```python
from build123d import *

# Parameters (mm, degrees)
SZKIC1_W                    = 12.5
SZKIC1_H                    = 37
DODANIE_WYCI_GNI_CIE1_DEPTH = 9.9
SZKIC2_W                    = 6.3
SZKIC2_H                    = 23.2
WYTNIJ_WYCI_GNI_CIE1_DEPTH  = 9.9
SZKIC3_R                    = 2
SZKIC3_R_2                  = 3.65
DODANIE_WYCI_GNI_CIE2_DEPTH = 7.5
WYTNIJ_WYCI_GNI_CIE2_DEPTH  = 78.151879433
WYTNIJ_WYCI_GNI_CIE3_DEPTH  = 72.402310887
ESQUISSE2_W                 = 2.9
ESQUISSE2_H                 = 5.1
ENL_V_MAT_EXTRU_1_DEPTH     = 6.3
BOSS_EXTRU_2_START          = -2.5
ESQUISSE5_R                 = 3.65
BOSS_EXTRU_2_DEPTH          = 2.5
BOSS_EXTRU_3_DEPTH          = 37
ESQUISSE7_R                 = 1.1
BOSS_EXTRU_4_DEPTH          = 4.5
ESQUISSE8_R                 = 1.65
ESQUISSE8_R_2               = 1.1
ENL_V_MAT_EXTRU_2_DEPTH     = 2.3
BOSS_EXTRU_7_START          = 1.2
BOSS_EXTRU_7_DEPTH          = 1.2
ENL_V_MAT_EXTRU_3_DEPTH     = 75.421317511
ENL_V_MAT_EXTRU_4_DEPTH     = 75.088410025


with BuildPart() as part:
    # Szkic1 → Dodanie-wyciągnięcie1 (new body)
    with BuildSketch(Plane.XY):
        with Locations((-6.25, 18.5)):
            Rectangle(SZKIC1_W, SZKIC1_H)
    extrude(amount=DODANIE_WYCI_GNI_CIE1_DEPTH)

    # Szkic2 → Wytnij-wyciągnięcie1 (cut)
    with BuildSketch(Plane.XY.offset(9.9)):
        with Locations((-3.15, 18.5)):
            Rectangle(SZKIC2_W, SZKIC2_H)
    extrude(amount=-WYTNIJ_WYCI_GNI_CIE1_DEPTH, mode=Mode.SUBTRACT)

    # Szkic3 → Dodanie-wyciągnięcie2 (add)
    with BuildSketch(Plane.ZY.offset(12.5)):
        with BuildLine():
            Line((55.440769231, 18.25), (57.7, -4))
            ThreePointArc((57.7, -4), (51.55, -10.15), (45.4, -4))
            Line((45.4, -4), (45.4, 0))
            Line((45.4, 0), (7.4, 0))
            Line((7.4, 0), (7.4, 37))
            Line((7.4, 37), (9.9, 37))
            Line((9.9, 37), (55.440769231, 18.25))
        make_face()
        with Locations((51.55, 12.25)):
            Circle(SZKIC3_R, mode=Mode.SUBTRACT)
        with Locations((51.55, -4)):
            Circle(SZKIC3_R_2, mode=Mode.SUBTRACT)
    extrude(amount=DODANIE_WYCI_GNI_CIE2_DEPTH)

    # Szkic4 → Wytnij-wyciągnięcie2 (cut, through all)
    with BuildSketch(Plane(origin=(0, 37, 0), x_dir=(1, 0, 0), z_dir=(0, 1, 0))):
        Polygon((-17.5, -9.9), (-15, -7.4), (-20, -7.4), (-20, -9.9), align=None)
        Polygon((-20, -12.4), (-17.5, -9.9), (-20, -9.9), align=None)
        Polygon((-12.5, -9.9), (-13.964466094, -9.9), (-17.5, -13.435533906), (-17.5, -57.7), (-12.5, -57.7), (-12.5, -55.440769231), align=None)
    extrude(amount=-WYTNIJ_WYCI_GNI_CIE2_DEPTH, mode=Mode.SUBTRACT)

    # Szkic5 → Wytnij-wyciągnięcie3 (cut, through all)
    with BuildSketch(Plane.ZY.offset(20)):
        with BuildLine():
            Line((45.4, 16.307054303), (45.4, 6))
            ThreePointArc((45.4, 6), (45.107106781, 5.292893219), (44.4, 5))
            Line((44.4, 5), (18.4, 5))
            ThreePointArc((18.4, 5), (17.692893219, 5.292893219), (17.4, 6))
            Line((17.4, 6), (17.4, 27.011748322))
            ThreePointArc((17.4, 27.011748322), (17.843544103, 27.842625469), (18.780713669, 27.936441299))
            Line((18.780713669, 27.936441299), (44.780713669, 17.23174728))
            ThreePointArc((44.780713669, 17.23174728), (45.230877148, 16.8635102), (45.4, 16.307054303))
        make_face()
    extrude(amount=-WYTNIJ_WYCI_GNI_CIE3_DEPTH, mode=Mode.SUBTRACT)

    # Esquisse2 → Enlèv. mat.-Extru.1 (cut)
    with BuildSketch(Plane(origin=(0, 0, 0), x_dir=(0, 0, -1), z_dir=(1, 0, 0))):
        with Locations((-3.95, 32.65)):
            Rectangle(ESQUISSE2_W, ESQUISSE2_H)
        with Locations((-3.95, 4.35)):
            Rectangle(ESQUISSE2_W, ESQUISSE2_H)
    extrude(amount=-ENL_V_MAT_EXTRU_1_DEPTH, mode=Mode.SUBTRACT)

    # Esquisse5 → Boss.-Extru.2 (add)
    with BuildSketch(Plane(origin=(-17.5, 0, 0), x_dir=(0, 0, -1), z_dir=(1, 0, 0)).offset(BOSS_EXTRU_2_START)):
        with BuildLine():
            Line((-13.435533906, 0), (-13.435533906, 35.544353513))
            Line((-13.435533906, 35.544353513), (-55.440769231, 18.25))
            Line((-55.440769231, 18.25), (-57.7, -4))
            ThreePointArc((-57.7, -4), (-51.55, -10.15), (-45.4, -4))
            Line((-45.4, -4), (-45.4, 0))
            Line((-45.4, 0), (-13.435533906, 0))
        make_face()
        with Locations(Location((-51.55, -4, 0), (0, 0, 180))):
            Circle(ESQUISSE5_R, mode=Mode.SUBTRACT)
        with BuildLine():
            Line((-17.4, 6), (-17.4, 27.011748322))
            ThreePointArc((-17.4, 27.011748322), (-17.843544103, 27.842625469), (-18.780713669, 27.936441299))
            Line((-18.780713669, 27.936441299), (-44.780713669, 17.23174728))
            ThreePointArc((-44.780713669, 17.23174728), (-45.230877148, 16.8635102), (-45.4, 16.307054303))
            Line((-45.4, 16.307054303), (-45.4, 6))
            ThreePointArc((-45.4, 6), (-45.107106781, 5.292893219), (-44.4, 5))
            Line((-44.4, 5), (-18.4, 5))
            ThreePointArc((-18.4, 5), (-17.692893219, 5.292893219), (-17.4, 6))
        make_face(mode=Mode.SUBTRACT)
    extrude(amount=BOSS_EXTRU_2_DEPTH)

    # Esquisse6 → Boss.-Extru.3 (add)
    with BuildSketch(Plane(origin=(0, 37, 0), x_dir=(1, 0, 0), z_dir=(0, 1, 0))):
        Polygon((-12.5, -4.9), (-15, -7.4), (-12.5, -7.4), align=None)
    extrude(amount=-BOSS_EXTRU_3_DEPTH)

    # Esquisse7 → Boss.-Extru.4 (add)
    # profile 1 of 2: a face of its own
    with BuildSketch(Plane(origin=(0, 0, 0), x_dir=(0, 0, -1), z_dir=(1, 0, 0))):
        with BuildLine():
            Line((-9.9, 37), (0, 37))
            ThreePointArc((0, 37), (-4.95, 41.95), (-9.9, 37))
        make_face()
        with Locations(Location((-4.95, 39.475, 0), (0, 0, 90))):
            Circle(ESQUISSE7_R, mode=Mode.SUBTRACT)
    # profile 2 of 2: a face of its own
    with BuildSketch(Plane(origin=(0, 0, 0), x_dir=(0, 0, -1), z_dir=(1, 0, 0))):
        with BuildLine():
            Line((-9.9, 0), (0, 0))
            ThreePointArc((0, 0), (-4.95, -4.95), (-9.9, 0))
        make_face()
        with Locations(Location((-4.95, -2.475, 0), (0, 0, 270))):
            Circle(ESQUISSE7_R, mode=Mode.SUBTRACT)
    extrude(amount=-BOSS_EXTRU_4_DEPTH)

    # Esquisse8 → Enlèv. mat.-Extru.2 (cut)
    # profile 1 of 2: a face of its own
    with BuildSketch(Plane(origin=(0, 0, 0), x_dir=(0, 0, -1), z_dir=(1, 0, 0))):
        with Locations(Location((-4.95, 39.475, 0), (0, 0, 90))):
            Circle(ESQUISSE8_R)
        with Locations(Location((-4.95, 39.475, 0), (0, 0, 90))):
            Circle(ESQUISSE8_R_2, mode=Mode.SUBTRACT)
    # profile 2 of 2: a face of its own
    with BuildSketch(Plane(origin=(0, 0, 0), x_dir=(0, 0, -1), z_dir=(1, 0, 0))):
        with Locations(Location((-4.95, -2.475, 0), (0, 0, 90))):
            Circle(ESQUISSE8_R)
        with Locations(Location((-4.95, -2.475, 0), (0, 0, 90))):
            Circle(ESQUISSE8_R_2, mode=Mode.SUBTRACT)
    extrude(amount=-ENL_V_MAT_EXTRU_2_DEPTH, mode=Mode.SUBTRACT)

    # Esquisse9 → Boss.-Extru.7 (add)
    with BuildSketch(Plane.ZY.offset(20).offset(BOSS_EXTRU_7_START)):
        with BuildLine():
            Line((12.4, 35.970702498), (12.4, 0))
            Line((12.4, 0), (45.4, 0))
            Line((45.4, 0), (45.4, -4))
            ThreePointArc((45.4, -4), (51.55, -10.15), (57.7, -4))
            Line((57.7, -4), (55.440769231, 18.25))
            Line((55.440769231, 18.25), (12.4, 35.970702498))
        make_face()
        with BuildLine():
            Line((47.863295083, -3.313919205), (49.350089671, 12.369863153))
            ThreePointArc((49.350089671, 12.369863153), (51.55, 14.55), (53.749910329, 12.369863153))
            Line((53.749910329, 12.369863153), (55.236704917, -3.313919205))
            ThreePointArc((55.236704917, -3.313919205), (51.55, -7.75), (47.863295083, -3.313919205))
        make_face(mode=Mode.SUBTRACT)
        with BuildLine():
            Line((18.780713669, 27.936441299), (44.780713669, 17.23174728))
            ThreePointArc((44.780713669, 17.23174728), (45.230877148, 16.8635102), (45.4, 16.307054303))
            Line((45.4, 16.307054303), (45.4, 6))
            ThreePointArc((45.4, 6), (45.107106781, 5.292893219), (44.4, 5))
            Line((44.4, 5), (18.4, 5))
            ThreePointArc((18.4, 5), (17.692893219, 5.292893219), (17.4, 6))
            Line((17.4, 6), (17.4, 27.011748322))
            ThreePointArc((17.4, 27.011748322), (17.843544103, 27.842625469), (18.780713669, 27.936441299))
        make_face(mode=Mode.SUBTRACT)
    extrude(amount=-BOSS_EXTRU_7_DEPTH)

    # Esquisse10 → Enlèv. mat.-Extru.3 (cut, through all)
    with BuildSketch(Plane.XZ):
        Polygon((-19.2, 43.7), (-19.2, 15.135533906), (-17.5, 13.435533906), (-17.5, 45.4), align=None)
        Polygon((-21.2, 12.4), (-20, 12.4), (-21.2, 13.6), align=None)
    extrude(amount=-ENL_V_MAT_EXTRU_3_DEPTH, mode=Mode.SUBTRACT)

    # Esquisse11 → Enlèv. mat.-Extru.4 (cut, through all)
    with BuildSketch(Plane.ZY.offset(20)):
        with BuildLine():
            ThreePointArc((52.05, 8.05), (51.903553391, 8.403553391), (51.55, 8.55))
            Line((51.55, 8.55), (51.55, 7.55))
            ThreePointArc((51.55, 7.55), (51.903553391, 7.696446609), (52.05, 8.05))
        make_face()
        with BuildLine():
            Line((51.55, 7.55), (51.55, 8.55))
            ThreePointArc((51.55, 8.55), (51.05, 8.05), (51.55, 7.55))
        make_face()
        with BuildLine():
            ThreePointArc((52.65, 8.05), (52.327817459, 8.827817459), (51.55, 9.15))
            Line((51.55, 9.15), (51.55, 8.55))
            ThreePointArc((51.55, 8.55), (51.903553391, 8.403553391), (52.05, 8.05))
            ThreePointArc((52.05, 8.05), (51.903553391, 7.696446609), (51.55, 7.55))
            Line((51.55, 7.55), (51.55, 6.95))
            ThreePointArc((51.55, 6.95), (52.327817459, 7.272182541), (52.65, 8.05))
        make_face()
        with BuildLine():
            Line((51.55, 8.55), (51.55, 9.15))
            ThreePointArc((51.55, 9.15), (50.45, 8.05), (51.55, 6.95))
            Line((51.55, 6.95), (51.55, 7.55))
            ThreePointArc((51.55, 7.55), (51.05, 8.05), (51.55, 8.55))
        make_face()
        with BuildLine():
            ThreePointArc((51.55, 3.75), (50.45, 2.65), (51.55, 1.55))
            Line((51.55, 1.55), (51.55, 2.15))
            ThreePointArc((51.55, 2.15), (51.05, 2.65), (51.55, 3.15))
            Line((51.55, 3.15), (51.55, 3.75))
        make_face()
        with BuildLine():
            Line((51.55, 2.15), (51.55, 1.55))
            ThreePointArc((51.55, 1.55), (52.327817459, 1.872182541), (52.65, 2.65))
            ThreePointArc((52.65, 2.65), (52.327817459, 3.427817459), (51.55, 3.75))
            Line((51.55, 3.75), (51.55, 3.15))
            ThreePointArc((51.55, 3.15), (51.903553391, 3.003553391), (52.05, 2.65))
            ThreePointArc((52.05, 2.65), (51.903553391, 2.296446609), (51.55, 2.15))
        make_face()
        with BuildLine():
            ThreePointArc((51.55, 3.15), (51.05, 2.65), (51.55, 2.15))
            Line((51.55, 2.15), (51.55, 3.15))
        make_face()
        with BuildLine():
            Line((51.55, 3.15), (51.55, 2.15))
            ThreePointArc((51.55, 2.15), (51.903553391, 2.296446609), (52.05, 2.65))
            ThreePointArc((52.05, 2.65), (51.903553391, 3.003553391), (51.55, 3.15))
        make_face()
    extrude(amount=-ENL_V_MAT_EXTRU_4_DEPTH, mode=Mode.SUBTRACT)


solid = part.part
```
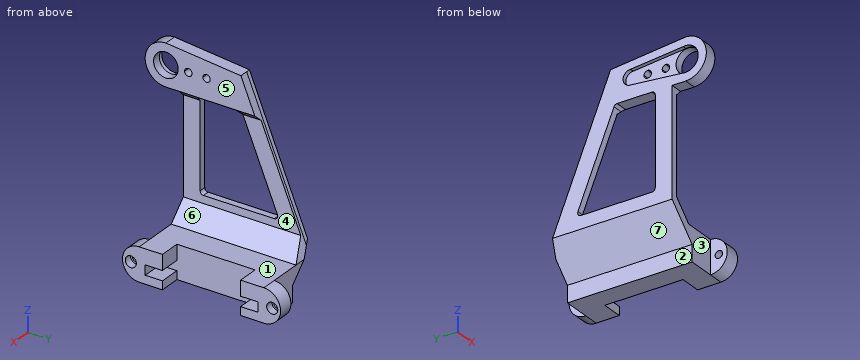
The model under review builds one solid part; all positions refer to its coordinate system, in mm. Face numbers are marked on the shaded views. A direction names the side the tool comes from. Round coordinates to 2 decimals unless told otherwise and drop trailing zeros. Order: outer loops, then holes, each group sorted by start corner. A loop starts at its lowest first (then second) coordinate and runs counter-clockwise, first axis right, second up.
Item 1: Add section A-A, the plane x = -3. State the section outline as (y, z) points (3 decimals).
Working result:
outline: (0, 0) - (6.9, 0) - (6.9, 2.5) - (1.8, 2.5) - (1.8, 5.4) - (6.9, 5.4) - (6.9, 9.9) - (0, 9.9) arc R4.95 ccw to start; (30.1, 0) - (37, 0) arc R4.95 ccw to (37, 9.9) - (30.1, 9.9) - (30.1, 5.4) - (35.2, 5.4) - (35.2, 2.5) - (30.1, 2.5) - close; hole circle Ø2.2 at (-2.475, 4.95); hole circle Ø2.2 at (39.475, 4.95)
Item 2: Machinability: for the marked faces 1, 2, 3 and 4, which of the approach directions +Z, -Z, +X, -X, +Y, -Y give a long, thin tool a straight path to every point of the face, cutting with its end or side? Answer none if there is none.
Working result:
face 1: +Z, +X, +Y, -Y
face 2: -Z, -X, +Y, -Y
face 3: -Z, -X, -Y
face 4: +X, +Y, -Y
Item 3: Add section C-C, the plane x = -8. State the section outline as (y, z) points.
Working result:
outline: (0, 0) - (37, 0) - (37, 9.9) - (0, 9.9) - close
Item 4: For pin 1 (3.5 mm diameter, centred on y = 14, z = 49.5, fed in from +X); pin 2 (1 mm diameter, centred on y = -3, z = 5.5, fed in from +X); pin 3 (3.5 mm diameter, centred on y = 39.475, z = 4.95, fed in from -X); pin 4 (6 mm diameter, centred on y = 3, z = 52, fed in from -X), all flat-tipped, find the tip position at first contact; note any pin that passes through.
Working result:
pin 1: stops at x = -17.5
pin 2: stops at x = -2.3
pin 3: stops at x = -4.5
pin 4: stops at x = -21.2
Item 5: Add section B-B, the plane z = 30. State the section outline as (x, y) points, and give its area (3 significant figures).
Working result:
outline: (-21.2, 0) - (-19.2, 0) - (-19.2, 5) - (-21.2, 5) - close; (-21.2, 23.32) - (-19.2, 23.32) - (-19.2, 28.72) - (-21.2, 28.72) - close
area: 20.8 mm2
Item 6: Draft analysis for pull direction Z (two halves, no side actions). For the marked faces 5, 6 and 7, state which applies: released by +Z, released by -Z, zero draft, split by the parting line, or undercut.
Working result:
face 5: zero draft
face 6: undercut
face 7: released by -Z
Item 7: To check wall thickness, follow probe 1 along Y at (x, z) = (-18.05, 51.55); probe 2 along Z at (x, y) = (-7.5, 33); probe 3 along Y at (x, z) = (-20.25, 20.5). State the ranges of each line that lie inside material, in increasing order.
Working result:
probe 1: y = -10.15 to -7.65, -0.35 to 1.55, 3.75 to 6.95, 9.15 to 19.85
probe 2: z = 0 to 9.9
probe 3: y = 0 to 5, 27.23 to 32.64
